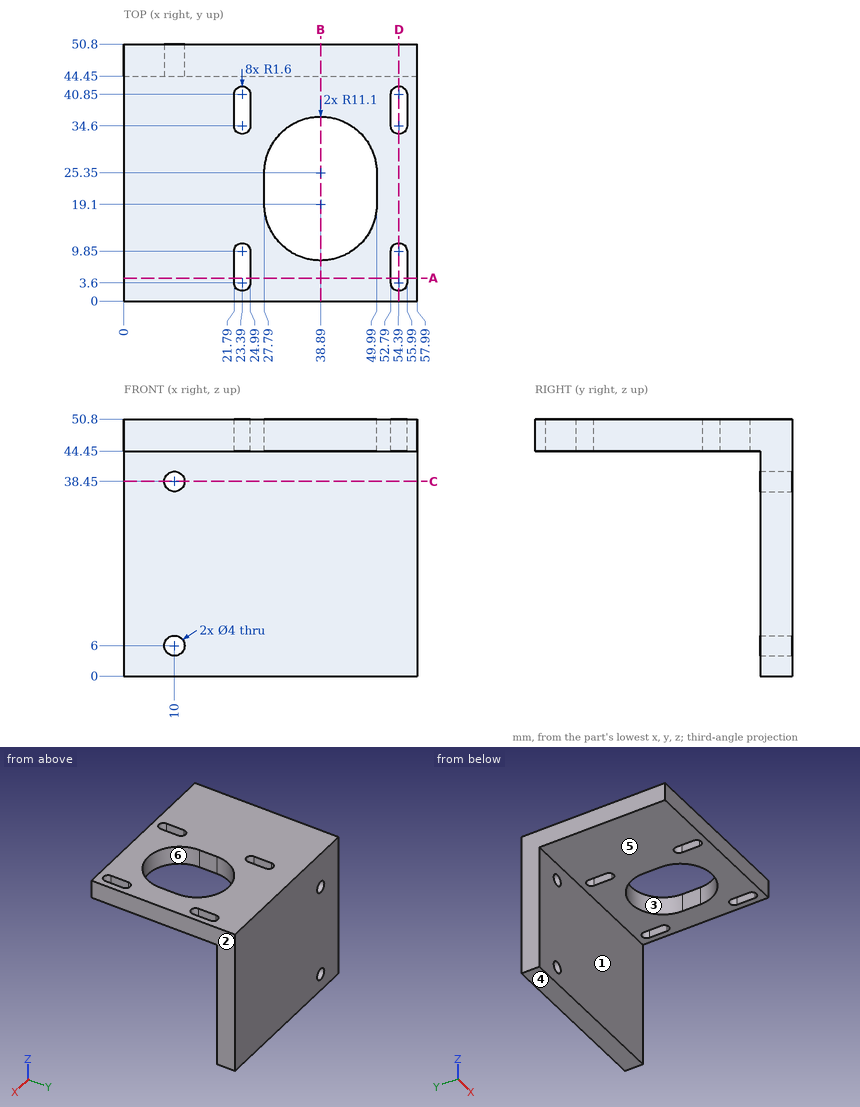
Print and shaded views of the part. All mm, measured from the part's lowest x, y and z. A direction names the side the tool comes from. Give positions to 0.01 mm unless a question says otherwise; leave off trailing zeros. Write each loop counter-clockwise with the first axis right and the second up, starting at its lowest first coordinate (ties: lowest second). Pieces come first, ordered by that corner, then holes. Notation, with made-up numbers: M -32.5,37.5 L -12.5,37.5 A33 cw -12.5,70.5 Z; hole C 77,-6 d2. An arc over 180 degrees is marked long. Use a Markdown table: item, result.
1) Cut at D-D (x = 54.39). List the corners of the cut face in (y, z), and give its area (3 significant figures).
Responses:
| item | result |
|---|---|
| outline | M 0,44.45 L 2,44.45 L 2,50.8 L 0,50.8 Z; M 11.45,44.45 L 33,44.45 L 33,50.8 L 11.45,50.8 Z; M 42.45,44.45 L 44.45,44.45 L 44.45,0 L 50.8,0 L 50.8,50.8 L 42.45,50.8 Z |
| area | 485 mm2 |
2) Tool access for the marked faces 4, 5 and 6: list every direction of +Z, -Z, +X, -X, +Y, -Y with a clear straight run to the whole face (end or side of a thin tool).
Responses:
| item | result |
|---|---|
| face 4 | -Z, +X, -X, +Y, -Y |
| face 5 | -Z, +X, -X, -Y |
| face 6 | +Z, -Z |
3) Cut at C-C (z = 38.45). List the corners of the cut face in (x, y).
Responses:
| item | result |
|---|---|
| outline | M 0,44.45 L 8,44.45 L 8,50.8 L 0,50.8 Z; M 12,44.45 L 57.99,44.45 L 57.99,50.8 L 12,50.8 Z |
4) Cut at B-B (x = 38.89). List the corners of the cut face in (y, z).
Responses:
| item | result |
|---|---|
| outline | M 0,44.45 L 8,44.45 L 8,50.8 L 0,50.8 Z; M 36.45,44.45 L 44.45,44.45 L 44.45,0 L 50.8,0 L 50.8,50.8 L 36.45,50.8 Z |
5) Pin check, flat tips, straight feed: pin 1 (5 mm diameter, centred on x = 23, y = 21, fed in from -Z); pin 2 (1.5 mm diameter, centred on x = 26, z = 7, fed in from -Y). Stop position of each tip, or through.
Responses:
| item | result |
|---|---|
| pin 1 | stops at z = 44.45 |
| pin 2 | stops at y = 44.45 |
6) Drill centre lines: line 1 (Z direction, x = 10, y = 49.75); line 2 (Y direction, x = 24.5, z = 44.5); line 3 (Z direction, x = 33.5, y = 2.5). Where is each one in solid material? Low to high. Write a range as from..to.
Responses:
| item | result |
|---|---|
| line 1 | z = 0..4, 8..36.45, 40.45..50.8 |
| line 2 | y = 0..2.45, 11..33.45, 42..50.8 |
| line 3 | z = 44.45..50.8 |
7) Pull direction X, two halves, no side cores. Call the marked faces 1, 2 and 3: +X half, -X half, draft (parallel to the pull), parting line (faces both ways), or undercut.
Responses:
| item | result |
|---|---|
| face 1 | draft |
| face 2 | +X half |
| face 3 | undercut |
8) Cut at A-A (y = 4.5). List the corners of the cut face in (x, z), and give its area (3 significant figures).
Responses:
| item | result |
|---|---|
| outline | M 0,44.45 L 21.79,44.45 L 21.79,50.8 L 0,50.8 Z; M 24.99,44.45 L 52.79,44.45 L 52.79,50.8 L 24.99,50.8 Z; M 55.99,44.45 L 57.99,44.45 L 57.99,50.8 L 55.99,50.8 Z |
| area | 328 mm2 |
